```python
from build123d import *

# Parameters (mm, degrees)
ESQUISSE2_W             = 200
ESQUISSE2_H             = 250
BOSS_EXTRU_1_DEPTH      = 10
ESQUISSE7_W             = 20
ESQUISSE7_H             = 10
ENL_V_MAT_EXTRU_2_DEPTH = 10
ENL_V_MAT_EXTRU_3_DEPTH = 10
ESQUISSE11_R            = 1.5
ESQUISSE11_R_2          = 1.37656202
ENL_V_MAT_EXTRU_4_DEPTH = 10
D_GAGEMENT_M31_D        = 3.4


with BuildPart() as part:
    # Esquisse2 → Boss.-Extru.1 (new body)
    with BuildSketch(Plane.XY):
        with Locations((100, -125)):
            Rectangle(ESQUISSE2_W, ESQUISSE2_H)
    extrude(amount=BOSS_EXTRU_1_DEPTH)

    # Esquisse7 → Enlèv. mat.-Extru.2 (cut)
    with BuildSketch(Plane(origin=(0, 0, 0), x_dir=(-1, 0, 0), z_dir=(0, 0, -1))):
        with Locations((-100, -125)):
            Rectangle(ESQUISSE7_W, ESQUISSE7_H)
    extrude(amount=-ENL_V_MAT_EXTRU_2_DEPTH, mode=Mode.SUBTRACT)

    # Esquisse10 → Enlèv. mat.-Extru.3 (cut)
    with BuildSketch(Plane(origin=(0, 0, 0), x_dir=(-1, 0, 0), z_dir=(0, 0, -1))):
        with BuildLine():
            Line((-70, -28.5), (-75, -28.5))
            ThreePointArc((-75, -28.5), (-78.5, -25), (-75, -21.5))
            Line((-75, -21.5), (-70, -21.5))
            ThreePointArc((-70, -21.5), (-66.5, -25), (-70, -28.5))
        make_face()
        with BuildLine():
            Line((-70, -228.5), (-75, -228.5))
            ThreePointArc((-75, -228.5), (-78.5, -225), (-75, -221.5))
            Line((-75, -221.5), (-70, -221.5))
            ThreePointArc((-70, -221.5), (-66.5, -225), (-70, -228.5))
        make_face()
        with BuildLine():
            Line((-130, -221.5), (-125, -221.5))
            ThreePointArc((-125, -221.5), (-121.5, -225), (-125, -228.5))
            Line((-125, -228.5), (-130, -228.5))
            ThreePointArc((-130, -228.5), (-133.5, -225), (-130, -221.5))
        make_face()
        with BuildLine():
            Line((-130, -21.5), (-125, -21.5))
            ThreePointArc((-125, -21.5), (-121.5, -25), (-125, -28.5))
            Line((-125, -28.5), (-130, -28.5))
            ThreePointArc((-130, -28.5), (-133.5, -25), (-130, -21.5))
        make_face()
    extrude(amount=-ENL_V_MAT_EXTRU_3_DEPTH, mode=Mode.SUBTRACT)

    # Esquisse11 → Enlèv. mat.-Extru.4 (cut)
    with BuildSketch(Plane(origin=(0, 0, 0), x_dir=(-1, 0, 0), z_dir=(0, 0, -1))):
        with Locations((-80, -190)):
            Circle(ESQUISSE11_R)
        with Locations((-120, -190)):
            Circle(ESQUISSE11_R)
        with Locations((-80, -60)):
            Circle(ESQUISSE11_R)
        with Locations((-120, -60)):
            Circle(ESQUISSE11_R_2)
    extrude(amount=-ENL_V_MAT_EXTRU_4_DEPTH, mode=Mode.SUBTRACT)

    # Dégagement M31 (through all)
    with Locations(Plane.XY.offset(10)):
        with Locations((18.5, -54.7), (54.5, -54.7), (18.545923706, -114.7), (54.5, -114.7), (145.5, -135.3), (181.5, -135.3), (145.5, -195.3), (181.5, -195.3)):
            Hole(D_GAGEMENT_M31_D / 2)


solid = part.part
```
Geometry: final body of the model. Coordinates: model frame, mm. A direction names the side the tool comes from. Coordinates: 2 decimals unless noted, no trailing zeros. Order: outer loops, then holes, each group sorted by start corner. A loop starts at its lowest first (then second) coordinate and runs counter-clockwise, first axis right, second up. Notation, with made-up numbers: (20, 43.25) - (77, 43.25) arc R25 cw to (77, 57.25) - close; hole circle Ø10 at (16, 11). An arc over 180 degrees is marked (long way). Write each question's results on one line, items separated by ' | '.
(1) Line query: line 1 (Y direction, x = 80, z = 5.25); line 2 (X direction, y = -195.3, z = 3.5); line 3 (X direction, y = -114.7, z = 4.75). Output: solid intervals per line, ascending. Write a range as [from, to].
Values found:
line 1: y = [-250, -191.5], [-188.5, -61.5], [-58.5, 0] | line 2: x = [0, 143.8], [147.2, 179.8], [183.2, 200] | line 3: x = [0, 16.85], [20.25, 52.8], [56.2, 200]
(2) Mould query, pull axis X, two halves, no side actions, for faces 3 (the face through (99, 0, 5)), 4 (the face through (0, -127, 5)), 5 (the face through (90, -125, 5)). Classes: +X half, -X half, draft (parallel to the pull), parting line (faces both ways), or undercut.
Values found:
face 3: draft | face 4: -X half | face 5: undercut
(3) Set-up query: faces 1 (the face through (121.5, -224.9, 4.9)), 2 (the face through (99, -250, 5)). Return all of +Z, -Z, +X, -X, +Y, -Y with unobstructed straight access to the full face (end or side cutting, diameter ignored); none if empty.
Values found:
face 1: +Z, -Z | face 2: +Z, -Z, +X, -X, -Y
(4) Section query A-A, the plane y = -25. Return the cut outline in (x, z), plus the area to 3 significant figures.
Values found:
outline: (0, 0) - (66.5, 0) - (66.5, 10) - (0, 10) - close; (78.5, 0) - (121.5, 0) - (121.5, 10) - (78.5, 10) - close; (133.5, 0) - (200, 0) - (200, 10) - (133.5, 10) - close | area: 1,760 mm²
(5) First-contact query: pin 1 Ø2.5 at (x, y) = (80, -60) entering from -Z. Flat tip, straight axial feed; report the tip coordinate or a pass-through.
Values found:
pin 1: passes through
